```python
from build123d import *

# Parameters (mm, degrees)
F0_W           = 203.2
F0_H           = 203.2
F1_DEPTH       = 127
F2_W           = 152.4
F2_H           = 152.4
F3_DEPTH       = 76.2
F4_W           = 152.4
F4_H           = 152.4
F6_C1_SIZE2    = 87.9881810245
F6_C1_SIZE     = 50.8
F6_C2_SIZE2    = 87.9881810245
F6_C2_SIZE     = 50.8
F6_C3_SIZE2    = 50.8
F6_C3_SIZE     = 87.9881810245
F6_C4_SIZE2    = 87.9881810245
F6_C4_SIZE     = 50.8
F8_DEPTH       = 127
F10_R          = 6.35
F11_DEPTH      = 76.2
F15_R          = 6.35
F16_DEPTH      = 127
F17_R          = 6.35
F18_DEPTH      = 127
F19_R          = 6.35
F20_DEPTH      = 127
F21_R          = 19.05
F22_DEPTH      = 50.8
F22_DEPTH_BACK = 12.7


# Not quite as in the source:
# - an extrude whose draft closes it to a point is written as a loft to that point


with BuildPart() as f1:
    # F0 (on Top) → F1 (new body)
    with BuildSketch(Plane.XY):
        Rectangle(F0_W, F0_H)
    extrude(amount=F1_DEPTH)

    # F2 (on face) → F3 (cut)
    with BuildSketch(Plane.XY):
        Rectangle(F2_W, F2_H)
    extrude(amount=F3_DEPTH, mode=Mode.SUBTRACT)

    # F4 (on face) → F5 section 0
    with BuildSketch(Plane(origin=(0, 0, 76.2), x_dir=(1, 0, 0), z_dir=(0, 0, -1)), mode=Mode.PRIVATE) as f5_s0:
        Rectangle(F4_W, F4_H)
    loft([f5_s0.sketch, Vertex(0, 0, 120.1940905122)], ruled=True, mode=Mode.SUBTRACT)

    # F6: chamfer of 50.8 x 87.9881810245 on 4 edges, made by hand

    # F6_c1
    f6_c1_edges = [f1.edges().sort_by_distance(p)[0] for p in [
        (0, -101.6, 127),
    ]]
    f6_c1_side = f1.faces().sort_by_distance((0, -101.6, 125.984))[0]
    chamfer(f6_c1_edges, length=F6_C1_SIZE, length2=F6_C1_SIZE2, reference=f6_c1_side)

    # F6_c2
    f6_c2_edges = [f1.edges().sort_by_distance(p)[0] for p in [
        (-101.6, 43.9940905122, 127),
    ]]
    f6_c2_side = f1.faces().sort_by_distance((-101.6, 43.9940905122, 125.984))[0]
    chamfer(f6_c2_edges, length=F6_C2_SIZE, length2=F6_C2_SIZE2, reference=f6_c2_side)

    # F6_c3
    f6_c3_edges = [f1.edges().sort_by_distance(p)[0] for p in [
        (101.6, 43.9940905122, 127),
    ]]
    f6_c3_side = f1.faces().sort_by_distance((100.584, 43.9940905122, 127))[0]
    chamfer(f6_c3_edges, length=F6_C3_SIZE, length2=F6_C3_SIZE2, reference=f6_c3_side)

    # F6_c4
    f6_c4_edges = [f1.edges().sort_by_distance(p)[0] for p in [
        (0, 101.6, 127),
    ]]
    f6_c4_side = f1.faces().sort_by_distance((0, 101.6, 125.984))[0]
    chamfer(f6_c4_edges, length=F6_C4_SIZE, length2=F6_C4_SIZE2, reference=f6_c4_side)

    # F7 (on Top) → F8 (cut, through all)
    with BuildSketch(Plane.XY):
        with BuildLine():
            Line((-19.3939794208, -14.9038513603), (-55.3150039051, -50.8248758446))
            ThreePointArc((-55.3150039051, -50.8248758446), (-55.3150039051, -55.3150039051), (-50.8248758446, -55.3150039051))
            Line((-50.8248758446, -55.3150039051), (-14.9038513603, -19.3939794208))
            ThreePointArc((-14.9038513603, -19.3939794208), (-14.9038513603, -14.9038513603), (-19.3939794208, -14.9038513603))
        make_face()
        with BuildLine():
            Line((-55.3150039051, 50.8248758446), (-19.3939794208, 14.9038513603))
            ThreePointArc((-19.3939794208, 14.9038513603), (-14.9038513603, 14.9038513603), (-14.9038513603, 19.3939794208))
            Line((-14.9038513603, 19.3939794208), (-50.8248758446, 55.3150039051))
            ThreePointArc((-50.8248758446, 55.3150039051), (-55.3150039051, 55.3150039051), (-55.3150039051, 50.8248758446))
        make_face()
        with BuildLine():
            Line((50.8248758446, 55.3150039051), (14.9038513603, 19.3939794208))
            ThreePointArc((14.9038513603, 19.3939794208), (14.9038513603, 14.9038513603), (19.3939794208, 14.9038513603))
            Line((19.3939794208, 14.9038513603), (55.3150039051, 50.8248758446))
            ThreePointArc((55.3150039051, 50.8248758446), (55.3150039051, 55.3150039051), (50.8248758446, 55.3150039051))
        make_face()
        with BuildLine():
            Line((55.3150039051, -50.8248758446), (19.3939794208, -14.9038513603))
            ThreePointArc((19.3939794208, -14.9038513603), (14.9038513603, -14.9038513603), (14.9038513603, -19.3939794208))
            Line((14.9038513603, -19.3939794208), (50.8248758446, -55.3150039051))
            ThreePointArc((50.8248758446, -55.3150039051), (55.3150039051, -55.3150039051), (55.3150039051, -50.8248758446))
        make_face()
    extrude(amount=F8_DEPTH, mode=Mode.SUBTRACT)

    # F10 (on face) → F11 (cut)
    with BuildSketch(Plane(origin=(87.0857142857, -87.0857142857, -50.2789605854), x_dir=(0.755928946, 0.5669467095, 0.3273268354), z_dir=(0.6546536707, -0.6546536707, -0.377964473))):
        with Locations((22.3436848712, 59.1158335421)):
            Circle(F10_R)
    extrude(amount=-F11_DEPTH, mode=Mode.SUBTRACT)

    # F15 (on face) → F16 (cut)
    with BuildSketch(Plane(origin=(-87.0857142857, -87.0857142857, -50.2789605854), x_dir=(0.5669467095, -0.755928946, 0.3273268354), z_dir=(-0.6546536707, -0.6546536707, -0.377964473))):
        with Locations((22.0481136328, 59.221623296)):
            Circle(F15_R)
    extrude(amount=-F16_DEPTH, mode=Mode.SUBTRACT)

    # F17 (on face) → F18 (cut)
    with BuildSketch(Plane(origin=(-87.0857142857, 87.0857142857, -50.2789605854), x_dir=(-0.755928946, -0.5669467095, 0.3273268354), z_dir=(-0.6546536707, 0.6546536707, -0.377964473))):
        with Locations((22.3436848712, 59.1158335421)):
            Circle(F17_R)
    extrude(amount=-F18_DEPTH, mode=Mode.SUBTRACT)

    # F19 (on face) → F20 (cut)
    with BuildSketch(Plane(origin=(87.0857142857, 87.0857142857, -50.2789605854), x_dir=(-0.755928946, 0.5669467095, -0.3273268354), z_dir=(0.6546536707, 0.6546536707, -0.377964473))):
        with Locations((-22.3436848712, 59.1158335421)):
            Circle(F19_R)
    extrude(amount=-F20_DEPTH, mode=Mode.SUBTRACT)

    # F21 (on face) → F22 (join, two sides)
    with BuildSketch(Plane.XY.offset(127)) as f22_sk:
        Circle(F21_R)
    extrude(amount=F22_DEPTH)
    extrude(f22_sk.sketch, amount=-F22_DEPTH_BACK)


solid = f1.part
```
Part model, mm, in its own coordinate system. A direction names the side the tool comes from. Coordinates: 2 decimals unless noted, no trailing zeros. Order: outer loops, then holes, each group sorted by start corner. A loop starts at its lowest first (then second) coordinate and runs counter-clockwise, first axis right, second up. Notation, with made-up numbers: (-10, 61) - (31, 61) arc R24 cw to (31, 72) - close; hole circle Ø10 at (54, 69). An arc over 180 degrees is marked (long way). Return JSON: item names as keys, results as strings. Group by question number.
Item 1: Pull direction X, two halves, no side cores. Call faces 1 (the face through (91.878, -82.902, 17.589)), 2 (the face through (0, 0, 177.8)), 3 (the face through (-101.6, -1, 38)), 4 (the face through (55.27, -55.36, 95.17)): pulls with the +X half, pulls with the -X half, needs draft (parallel to the pull), parting line crosses it, or undercut.
Item 2: Cut at D-D (z = 95.5). List the corners of the cut face in (x, y) (3 decimals), plus the area to 3 significant figures.
Item 3: Cut at A-A (z = 69). List the corners of the cut face in (x, y).
Item 4: Drill centre lines: probe 1 along X at (y, z) = (20, 55); probe 2 along X at (y, z) = (81.5, 22.5). Where is each one in solid material? Low to high. Write a range as from..to.
Item 5: Pin check, flat tips, straight feed: pin 1 (3 mm diameter, centred on x = -13.5, z = 119, fed in from -Y); pin 2 (6 mm diameter, centred on x = 2, y = -2.5, fed in from -Z); pin 3 (8 mm diameter, centred on x = 29.5, y = -43, fed in from +Z). Stop position of each tip, or through.
Item 6: Cut at C-C (x = 0). List the corners of the cut face in (y, z), plus the area to 3 significant figures.
Item 7: Cut at B-B (x = 38.5). List the corners of the cut face in (y, z).
Item 8: Which spindle directions (+Z, -Z, +X, -X, +Y, -Y) get a long thin tool onto all of the face, cutting with end or side? Do faces 5 (the face through (-1, 101.6, 38)), 6 (the face through (-32.61, 37.1, 105.71)), 7 (the face through (76.2, -1, 38)). Say none if no direction does.
Check values:
{
 "1": {"face 1": "undercut", "face 2": "needs draft", "face 3": "pulls with the -X half", "face 4": "undercut"},
 "2": {"outline": "(-68.171, -68.171) - (68.171, -68.171) - (68.171, 68.171) - (-68.171, 68.171) - close; hole (-55.315, -50.825) arc R3.175 ccw to (-50.825, -55.315) - (-38.281, -42.771) - (38.281, -42.771) - (50.825, -55.315) arc R3.175 ccw to (55.315, -50.825) - (42.771, -38.281) - (42.771, 38.281) - (55.315, 50.825) arc R3.175 ccw to (50.825, 55.315) - (38.281, 42.771) - (-38.281, 42.771) - (-50.825, 55.315) arc R3.175 ccw to (-55.315, 50.825) - (-42.771, 38.281) - (-42.771, -38.281) - close", "area": "10,800 mm2"},
 "3": {"outline": "(-101.6, -101.6) - (101.6, -101.6) - (101.6, 101.6) - (-101.6, 101.6) - close; hole (-76.2, -76.2) - (76.2, -76.2) - (76.2, 76.2) - (-76.2, 76.2) - close"},
 "4": {"probe 1": "x = -101.6..-76.2, 76.2..101.6", "probe 2": "x = -101.6..-89.21, -72.67..72.67, 89.21..101.6"},
 "5": {"pin 1": "stops at y = -30.07", "pin 2": "stops at z = 114.3", "pin 3": "stops at z = 112.34"},
 "6": {"outline": "(-101.6, 0) - (-76.2, 0) - (-76.2, 76.2) - (-10.21, 114.3) - (10.21, 114.3) - (76.2, 76.2) - (76.2, 0) - (101.6, 0) - (101.6, 76.2) - (19.05, 123.86) - (19.05, 177.8) - (-19.05, 177.8) - (-19.05, 123.86) - (-101.6, 76.2) - close", "area": "8,380 mm2"},
 "7": {"outline": "(-101.6, 0) - (-76.2, 0) - (-76.2, 76.2) - (-42.99, 95.37) - (-42.99, 110.04) - (-101.6, 76.2) - close; (-34.01, 97.97) - (34.01, 97.97) - (34.01, 112.63) - (-34.01, 112.63) - close; (42.99, 95.37) - (76.2, 76.2) - (76.2, 0) - (101.6, 0) - (101.6, 76.2) - (42.99, 110.04) - close"},
 "8": {"face 5": "+Z, -Z, +X, -X, +Y", "face 6": "+Z, -Z", "face 7": "-Z"}
}
